from build123d import *

# Parameters (mm, degrees)
SKETCH1_W                = 19.43
SKETCH1_H                = 15.62
BOSS_EXTRUDE1_DEPTH      = 2.29
SKETCH5_W                = 15.25
SKETCH5_H                = 12.7
BOSS_EXTRUDE2_DEPTH      = 7.11
SKETCH6_W                = 12.7
SKETCH6_H                = 6
BOSS_EXTRUDE3_DEPTH      = 7.11
SKETCH7_W                = 0.76
SKETCH7_H                = 2.03
BOSS_EXTRUDE4_DEPTH      = 3.94
BOSS_EXTRUDE5_DEPTH      = 5.715
BOSS_EXTRUDE5_DEPTH_BACK = 5.715
SKETCH8_W                = 2.36
SKETCH8_H                = 17.09


with BuildPart() as part:
    # Sketch1 → Boss-Extrude1 (new body)
    with BuildSketch(Plane(origin=(0, 0, 0), x_dir=(1, 0, 0), z_dir=(0, 1, 0))):
        Rectangle(SKETCH1_W, SKETCH1_H)
    extrude(amount=BOSS_EXTRUDE1_DEPTH)

    # Sketch5 → Boss-Extrude2 (add)
    with BuildSketch(Plane.XZ):
        Rectangle(SKETCH5_W, SKETCH5_H)
    extrude(amount=BOSS_EXTRUDE2_DEPTH)

    # Sketch6 → Boss-Extrude3 (add)
    with BuildSketch(Plane.XZ.offset(7.11)):
        Rectangle(SKETCH6_W, SKETCH6_H)
    extrude(amount=BOSS_EXTRUDE3_DEPTH)

    # Sketch7 → Boss-Extrude4 (add)
    with BuildSketch(Plane.XZ.offset(14.22)):
        Rectangle(SKETCH7_W, SKETCH7_H)
        with Locations((-4.7, 0)):
            Rectangle(SKETCH7_W, SKETCH7_H)
        with Locations((4.7, 0)):
            Rectangle(SKETCH7_W, SKETCH7_H)
    extrude(amount=BOSS_EXTRUDE4_DEPTH)

    # Sketch8 → Boss-Extrude5 (add, two sides: drawn at the far end of the back side and taken through both)
    with BuildSketch(Plane.XY.offset(-BOSS_EXTRUDE5_DEPTH_BACK)):
        with Locations((0, 5.545)):
            Rectangle(SKETCH8_W, SKETCH8_H)
    extrude(amount=BOSS_EXTRUDE5_DEPTH + BOSS_EXTRUDE5_DEPTH_BACK)


solid = part.part
Can you work these out from the model? Positions are in its coordinate system, mm. A direction names the side the tool comes from. Give positions to 0.01 mm unless a question says otherwise; leave off trailing zeros. Order: outer loops, then holes, each group sorted by start corner. A loop starts at its lowest first (then second) coordinate and runs counter-clockwise, first axis right, second up. Notation, with made-up numbers: (75.25, 65) - (112.25, 65) arc R12 ccw to (112.25, 69) - close; hole circle Ø6 at (-9.75, 44.25). An arc over 180 degrees is marked (long way). Write each question's results on one line, items separated by ' | '.
1) Please list where these lines run through material, in increasing order: line 1 along Y through (x, z) = (1, 2.25); line 2 along Y through (x, z) = (5.25, 5); line 3 along X through (y, z) = (9, 1.5). Write a range as [from, to].
Final values:
line 1: y = [-14.22, 14.09] | line 2: y = [-7.11, 2.29] | line 3: x = [-1.18, 1.18]
2) If we mould it in two halves opening along X, with no side actions, what happens to faces 6 (the face through (0.38, -16, 0)), 7 (the face through (0, 1, 7.81)), 8 (the face through (-9.715, 1, 0))? For each: pulls with the +X half, pulls with the -X half, needs draft (parallel to the pull), parting line crosses it, or undercut.
Final values:
face 6: undercut | face 7: needs draft | face 8: pulls with the -X half
3) Suppose I cut it at A-A, the plane x = 0. Write out the boundary of the cut face in (y, z) (3 decimals).
Final values:
outline: (-18.16, -1.015) - (-14.22, -1.015) - (-14.22, -3) - (-7.11, -3) - (-7.11, -6.35) - (0, -6.35) - (0, -7.81) - (2.29, -7.81) - (2.29, -5.715) - (14.09, -5.715) - (14.09, 5.715) - (2.29, 5.715) - (2.29, 7.81) - (0, 7.81) - (0, 6.35) - (-7.11, 6.35) - (-7.11, 3) - (-14.22, 3) - (-14.22, 1.015) - (-18.16, 1.015) - close
4) Suppose I cut it at D-D, the plane x = 2.5. Write out the boundary of the cut face in (y, z).
Final values:
outline: (-14.22, -3) - (-7.11, -3) - (-7.11, -6.35) - (0, -6.35) - (0, -7.81) - (2.29, -7.81) - (2.29, 7.81) - (0, 7.81) - (0, 6.35) - (-7.11, 6.35) - (-7.11, 3) - (-14.22, 3) - close
5) On a 3-axis mill with a long thin cutter (end or side, diameter ignored), from which of +Z, -Z, +X, -X, +Y, -Y can I reach the whole of each face in a straight line? I mean faces 1 (the face through (0, -11, -3)), 2 (the face through (6.35, -11, 0)), 3 (the face through (0, -4, 6.35)), 4 (the face through (-1.18, 8, 0)), 5 (the face through (0, 8, -5.715)). Say none if no direction works.
Final values:
face 1: -Z, +X, -X, -Y | face 2: +Z, -Z, +X, -Y | face 3: +Z, +X, -X, -Y | face 4: +Z, -Z, -X, +Y | face 5: -Z, +X, -X, +Y
6) Suppose I cut it at B-B, the plane z = -0.25. Write out the boundary of the cut face in (x, y) (3 decimals).
Final values:
outline: (-9.715, 0) - (-7.625, 0) - (-7.625, -7.11) - (-6.35, -7.11) - (-6.35, -14.22) - (-5.08, -14.22) - (-5.08, -18.16) - (-4.32, -18.16) - (-4.32, -14.22) - (-0.38, -14.22) - (-0.38, -18.16) - (0.38, -18.16) - (0.38, -14.22) - (4.32, -14.22) - (4.32, -18.16) - (5.08, -18.16) - (5.08, -14.22) - (6.35, -14.22) - (6.35, -7.11) - (7.625, -7.11) - (7.625, 0) - (9.715, 0) - (9.715, 2.29) - (1.18, 2.29) - (1.18, 14.09) - (-1.18, 14.09) - (-1.18, 2.29) - (-9.715, 2.29) - close
7) Suppose I cut it at C-C, the plane y = -0.5. Write out the boundary of the cut face in (x, z) (3 decimals), then the cut area to 3 significant figures.
Final values:
outline: (-7.625, -6.35) - (7.625, -6.35) - (7.625, 6.35) - (-7.625, 6.35) - close | area: 194 mm^2
8) I'm going to push flat-ended pins straight in: pin 1 Ø1.5 at (x, y) = (-2.5, -9.5) entering from +Z; pin 2 Ø5 at (y, z) = (-11, 1.5) entering from +X; pin 3 Ø1.9 at (x, y) = (0, 7.5) entering from +Z (3 decimals). Where does each tip first touch, or does it pass through?
Final values:
pin 1: stops at z = 3 | pin 2: stops at x = 6.35 | pin 3: stops at z = 5.715
